Could you check a few things on this model? Use its own coordinates, in mm. Coordinates: 2 decimals unless noted, no trailing zeros. Loops run counter-clockwise (first coordinate to the right, second up) from the corner with the lowest first, then second, coordinate; pieces in that order, holes last. Notation, with made-up numbers: (44, -28.5) - (98, -28.5) arc R26 cw to (98, -11.5) - close; hole circle Ø8 at (36, 4). An arc over 180 degrees is marked (long way). One line per item, written item: value. Start each with the question number.
(1) If I drill on line 1 along Y through (x, z) = (163.5, 1.25); line 2 along X through (y, z) = (5, 0.7); line 3 along X through (y, z) = (52, 0.2), over which ranges is the centre line in solid material (lowest first)? Write a range as from..to.
(2) If we section it at B-B on y = 77: Write out the boundary of the cut face in (x, z).
(3) If we section it at A-A on z = 1.55: Count the separate pieces of the cut face and the enclosed holes in it, then the cut area to 3 significant figures.
(4) I'm going to push a flat-ended pin straight in: P1, Ø0.6, axis at x = 165, z = 1, coming from the +Y side. Where does the tip first touch, or does it pass through?
(5) If we section it at C-C on y = 37: Write out the boundary of the cut face in (x, z).
```python
from build123d import *

# Parameters (mm, degrees)
PAD_DEPTH = 2


with BuildPart() as part:
    # Sketch → Pad (new body)
    with BuildSketch(Plane.XY):
        Polygon((157.033, 67.5042), (171.483, 67.5042), (171.533, 60.1542), (159.683, 60.2542), (159.783, 49.4542), (159.683, 15.2042), (171.983, 15.1542), (171.983, 0.454206), (171.883, 0.404206), (0.133118, 0.321209), (0.133118, 89.0212), (120.783, 89.0712), (120.783, 70.8212), (157.033, 70.7542), align=None)
        Polygon((77.4245, 27.1042), (77.291943, 26.437791), (76.914453, 25.872837), (76.349499, 25.495347), (75.68309, 25.36279), (75.016681, 25.495347), (74.451727, 25.872837), (74.074237, 26.437791), (73.94168, 27.1042), (74.078529, 27.782035), (74.451727, 28.335563), (75.005255, 28.708761), (75.68309, 28.84561), (76.349499, 28.713053), (76.914453, 28.335563), (77.291943, 27.770609), align=None, mode=Mode.SUBTRACT)
        Polygon((82.4745, 8.40421), (82.341943, 7.737801), (81.964453, 7.172847), (81.399499, 6.795357), (80.73309, 6.6628), (80.066681, 6.795357), (79.501727, 7.172847), (79.124237, 7.737801), (78.99168, 8.40421), (79.124237, 9.070619), (79.501727, 9.635573), (80.066681, 10.013063), (80.73309, 10.14562), (81.399499, 10.013063), (81.964453, 9.635573), (82.341943, 9.070619), align=None, mode=Mode.SUBTRACT)
        Polygon((28.4245, 27.1542), (28.291943, 26.487791), (27.914453, 25.922837), (27.349499, 25.545347), (26.68309, 25.41279), (26.005255, 25.549639), (25.451727, 25.922837), (25.078529, 26.476365), (24.94168, 27.1542), (25.078529, 27.832035), (25.451727, 28.385563), (26.005255, 28.758761), (26.68309, 28.89561), (27.349499, 28.763053), (27.914453, 28.385563), (28.291943, 27.820609), align=None, mode=Mode.SUBTRACT)
        Polygon((120.025, 6.05421), (119.892443, 5.387801), (119.514953, 4.822847), (118.949999, 4.445357), (118.28359, 4.3128), (117.617181, 4.445357), (117.052227, 4.822847), (116.674737, 5.387801), (116.54218, 6.05421), (116.674737, 6.720619), (117.052227, 7.285573), (117.617181, 7.663063), (118.28359, 7.79562), (118.949999, 7.663063), (119.514953, 7.285573), (119.892443, 6.720619), align=None, mode=Mode.SUBTRACT)
        Polygon((169.033, 6.00421), (168.900443, 5.337801), (168.522953, 4.772847), (167.957999, 4.395357), (167.29159, 4.2628), (166.613758, 4.399652), (166.060234, 4.772851), (165.687038, 5.326377), (165.55019, 6.00421), (165.687038, 6.682043), (166.060234, 7.235569), (166.613758, 7.608768), (167.29159, 7.74562), (167.957999, 7.613063), (168.522953, 7.235573), (168.900443, 6.670619), align=None, mode=Mode.SUBTRACT)
        Polygon((82.4745, 51.0956), (82.341943, 50.429191), (81.964453, 49.864237), (81.399499, 49.486747), (80.73309, 49.35419), (80.066681, 49.486747), (79.501727, 49.864237), (79.124237, 50.429191), (78.99168, 51.0956), (79.124237, 51.762009), (79.501727, 52.326963), (80.066681, 52.704453), (80.73309, 52.83701), (81.399499, 52.704453), (81.964453, 52.326963), (82.341943, 51.762009), align=None, mode=Mode.SUBTRACT)
        Polygon((169.033, 64.0542), (168.900443, 63.387791), (168.522953, 62.822837), (167.957999, 62.445347), (167.29159, 62.31279), (166.613758, 62.449642), (166.060234, 62.822841), (165.687038, 63.376367), (165.55019, 64.0542), (165.687038, 64.732033), (166.060234, 65.285559), (166.613758, 65.658758), (167.29159, 65.79561), (167.957999, 65.663053), (168.522953, 65.285563), (168.900443, 64.720609), align=None, mode=Mode.SUBTRACT)
        Polygon((28.4245, 85.1042), (28.28765, 84.42637), (27.914453, 83.872847), (27.36093, 83.49965), (26.6831, 83.3628), (26.00527, 83.49965), (25.451747, 83.872847), (25.07855, 84.42637), (24.9417, 85.1042), (25.07855, 85.78203), (25.451747, 86.335553), (26.00527, 86.70875), (26.6831, 86.8456), (27.36093, 86.70875), (27.914453, 86.335553), (28.28765, 85.78203), align=None, mode=Mode.SUBTRACT)
        Polygon((5.57453, 50.9456), (5.437678, 50.267768), (5.064479, 49.714244), (4.510953, 49.341048), (3.83312, 49.2042), (3.155287, 49.341048), (2.601761, 49.714244), (2.228562, 50.267768), (2.09171, 50.9456), (2.228562, 51.623432), (2.601761, 52.176956), (3.155287, 52.550152), (3.83312, 52.687), (4.510953, 52.550152), (5.064479, 52.176956), (5.437678, 51.623432), align=None, mode=Mode.SUBTRACT)
        Polygon((5.52453, 8.49562), (5.391973, 7.829211), (5.014483, 7.264257), (4.449529, 6.886767), (3.78312, 6.75421), (3.116711, 6.886767), (2.551757, 7.264257), (2.174267, 7.829211), (2.04171, 8.49562), (2.178567, 9.173446), (2.551768, 9.726963), (3.105292, 10.100154), (3.78312, 10.237), (4.460948, 10.100154), (5.014472, 9.726963), (5.387673, 9.173446), align=None, mode=Mode.SUBTRACT)
    extrude(amount=PAD_DEPTH)


solid = part.part
```
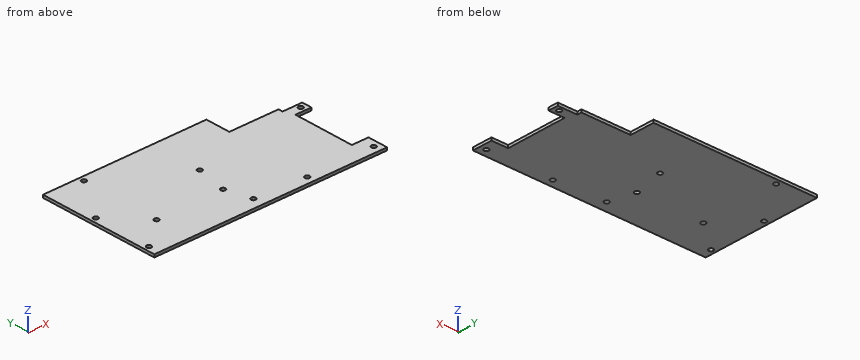
Values:
1. line 1: y = 0.4..15.19, 60.22..67.5
1. line 2: x = 0.13..116.93, 119.63..165.91, 168.67..171.98
1. line 3: x = 0.13..2.48, 5.18..79.28, 82.18..159.76
2. outline: (0.13, 0) - (120.78, 0) - (120.78, 2) - (0.13, 2) - close
3. separate pieces: 1
3. enclosed holes: 10
3. area: 13,600 mm2
4. P1: stops at y = 67.5
5. outline: (0.13, 0) - (159.75, 0) - (159.75, 2) - (0.13, 2) - close
